```python
from build123d import *

# Parameters (mm, degrees)
SKETCH1_R           = 4
BOSS_EXTRUDE1_DEPTH = 53
SKETCH2_R           = 5.5
BOSS_EXTRUDE2_DEPTH = 3
FILLET1_R           = 2
SKETCH4_W           = 0.5
SKETCH4_H           = 1


with BuildPart() as part:
    # Sketch1 → Boss-Extrude1 (new body)
    with BuildSketch(Plane(origin=(0, 0, 0), x_dir=(0, 0, -1), z_dir=(1, 0, 0))):
        Circle(SKETCH1_R)
    extrude(amount=BOSS_EXTRUDE1_DEPTH)

    # Sketch2 → Boss-Extrude2 (add)
    with BuildSketch(Plane.ZY):
        Circle(SKETCH2_R)
    extrude(amount=BOSS_EXTRUDE2_DEPTH)

    # Fillet1
    fillet1_edges = [part.edges().sort_by_distance(p)[0] for p in [
        (-3, 0, -5.5),
    ]]
    fillet(fillet1_edges, radius=FILLET1_R)

    # Sketch4 → Cut-Revolve1 (revolve, cut)
    with BuildSketch(Plane.XY, mode=Mode.PRIVATE) as cut_revolve1_sk:
        with Locations((48.5, 4)):
            Rectangle(SKETCH4_W, SKETCH4_H)
    revolve(cut_revolve1_sk.sketch.rotate(Axis((0, 0, 0), (1, 0, 0)), 90), axis=Axis((0, 0, 0), (1, 0, 0)), mode=Mode.SUBTRACT)


solid = part.part
```
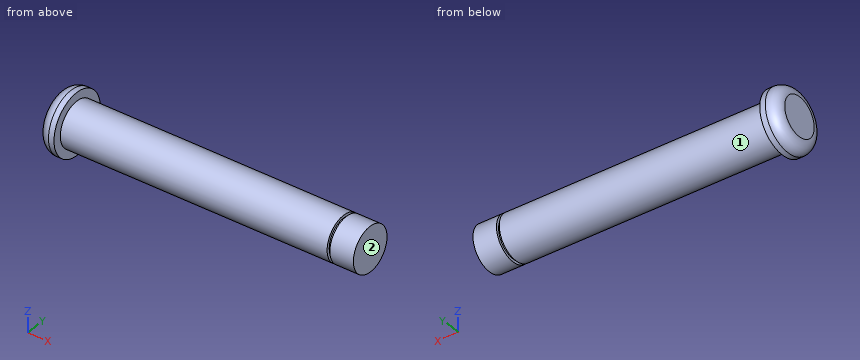
The model under review builds one solid part; all positions refer to its coordinate system, in mm. Face numbers are marked on the shaded views. A direction names the side the tool comes from. Round coordinates to 2 decimals unless told otherwise and drop trailing zeros. Order: outer loops, then holes, each group sorted by start corner. A loop starts at its lowest first (then second) coordinate and runs counter-clockwise, first axis right, second up.
(1) Take a section at A-A, the plane y = 0. State the section outline as (x, z) points.
Working result:
outline: (-3, -3.5) arc R2 ccw to (-1, -5.5) - (0, -5.5) - (0, -4) - (48.25, -4) - (48.25, -3.5) - (48.75, -3.5) - (48.75, -4) - (53, -4) - (53, 4) - (48.75, 4) - (48.75, 3.5) - (48.25, 3.5) - (48.25, 4) - (0, 4) - (0, 5.5) - (-1, 5.5) arc R2 ccw to (-3, 3.5) - close
(2) For P1, Ø2, axis at x = 4, z = 3.5, coming from the -Y side; P2, Ø5, axis at x = 40, y = 3.5, coming from the -Z side; P3, Ø1, axis at x = 39.5, y = 1.5, coming from the +Z side; P4, Ø4, axis at y = -0.5, z = -4, coming from the +X side, all flat-tipped, find the tip position at first contact; note any pin that passes through.
Working result:
P1: stops at y = -3.12
P2: stops at z = -3.87
P3: stops at z = 3.87
P4: stops at x = 53
(3) Tool access review of the marked faces 1 and 2: name each direction out of +Z, -Z, +X, -X, +Y, -Y from which nothing blocks a thin tool from reaching the whole face with its end or side.
Working result:
face 1: +X
face 2: +Z, -Z, +X, +Y, -Y
(4) Take a section at C-C, the plane x = 28.5. State the section outline as (y, z) points.
Working result:
outline: circle Ø8 at (0, 0)
(5) Wall thickness on L1, parallel to X at y = -1, z = 3.75; L2, parallel to Y at x = 40, z = -1.25; L3, parallel to Z at x = 11.5, y = 2.25: over which ranges is each line inside the solid? List them lowest first.
Working result:
L1: x = -2.96 to 48.25, 48.75 to 53
L2: y = -3.8 to 3.8
L3: z = -3.31 to 3.31
